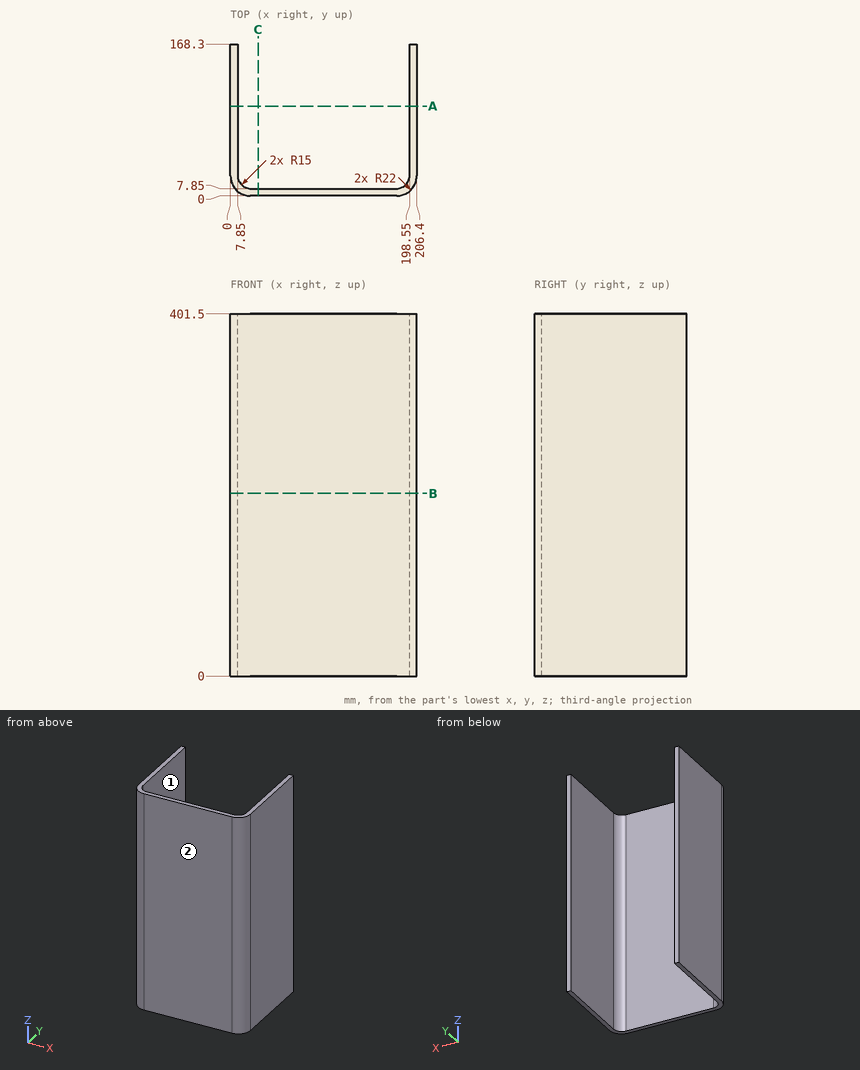
Design review of the part shown in the three views and the two pictorial views. Dimensions are in mm from the part's minimum x, y and z. A direction names the side the tool comes from. Coordinates: 2 decimals unless noted, no trailing zeros. Write each loop counter-clockwise with the first axis right and the second up, starting at its lowest first coordinate (ties: lowest second). Pieces come first, ordered by that corner, then holes.
1) We need section A-A on y = 99.5. State the section outline as (x, z) points.
2) We need section B-B on z = 202.5. State the section outline as (x, y) points.
3) Clearance check with a flat-ended pin moving along its axis: pin 1 Ø8 at (x, z) = (135.5, 73.5) entering from +Y. State where the tip first meets the part, or that it passes through.
4) We need section C-C on x = 30.5. State the section outline as (y, z) points, then the cut area to 3 significant figures.
5) Machinability: for the marked faces 1 and 2, which of the approach directions +Z, -Z, +X, -X, +Y, -Y give a long, thin tool a straight path to every point of the face, cutting with its end or side? Answer none if there is none.
6) To check wall thickness, follow probe 1 along X at (y, z) = (74, 102); probe 2 along Y at (x, z) = (121.5, 231); probe 3 along X at (y, z) = (9, 31). State the ranges of each line that lie inside material, in increasing order.
Answer list:
1. outline: (0, 0) - (7.85, 0) - (7.85, 401.5) - (0, 401.5) - close; (198.55, 0) - (206.4, 0) - (206.4, 401.5) - (198.55, 401.5) - close
2. outline: (0, 22) arc R22 ccw to (22, 0) - (184.4, 0) arc R22 ccw to (206.4, 22) - (206.4, 168.3) - (198.55, 168.3) - (198.55, 22.85) arc R15 cw to (183.55, 7.85) - (22.85, 7.85) arc R15 cw to (7.85, 22.85) - (7.85, 168.3) - (0, 168.3) - close
3. pin 1: stops at y = 7.85
4. outline: (0, 0) - (7.85, 0) - (7.85, 401.5) - (0, 401.5) - close
4. area: 3,150 mm2
5. face 1: +Z, -Z, +Y
5. face 2: +Z, -Z, +X, -X, -Y
6. probe 1: x = 0 to 7.85, 198.55 to 206.4
6. probe 2: y = 0 to 7.85
6. probe 3: x = 4.25 to 17.09, 189.31 to 202.15
